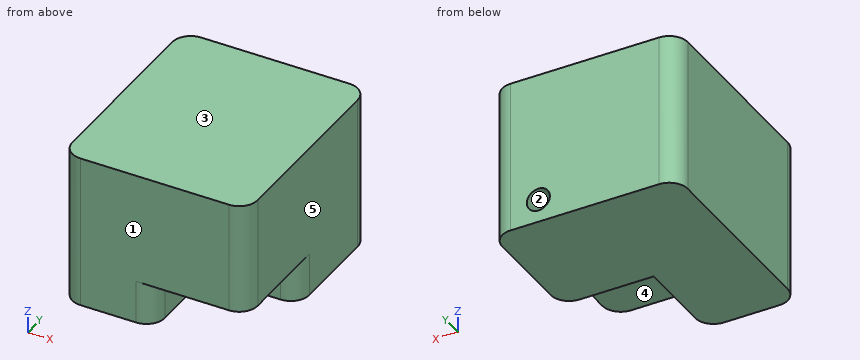
```python
from build123d import *

# Parameters (mm, degrees)
F0_W     = 30
F0_H     = 25
F1_DEPTH = 35
F2_W     = 15
F2_H     = 7
F3_DEPTH = 15
F4_R     = 1.865436
F5_DEPTH = 20.001
F6_R     = 3


with BuildPart() as f1:
    # F0 (on Front) → F1 (new body)
    with BuildSketch(Plane.XZ):
        with Locations((15, -12.5)):
            Rectangle(F0_W, F0_H)
    extrude(amount=F1_DEPTH)

    # F2 (on face) → F3 (cut)
    with BuildSketch(Plane.XZ.offset(35)):
        with Locations((22.5, -21.5)):
            Rectangle(F2_W, F2_H)
    extrude(amount=-F3_DEPTH, mode=Mode.SUBTRACT)

    # F4 (on face) → F5 (cut, through all)
    with BuildSketch(Plane.XZ.offset(20)):
        with Locations((22.5, -21.223269)):
            Circle(F4_R)
    extrude(amount=-F5_DEPTH, mode=Mode.SUBTRACT)

    # F6
    f6_edges = [f1.edges().sort_by_distance(p)[0] for p in [
        (0, -35, -12.5),
        (15, -35, -21.5),
        (30, 0, -12.5),
        (30, -35, -9),
        (30, -20, -21.5),
        (0, 0, -12.5),
    ]]
    fillet(f6_edges, radius=F6_R)


solid = f1.part
```
CAD build for the part. Positions are in the model's coordinates, mm. Face numbers are marked on the shaded views. A direction names the side the tool comes from. Coordinates: 2 decimals unless noted, no trailing zeros. Order: outer loops, then holes, each group sorted by start corner. A loop starts at its lowest first (then second) coordinate and runs counter-clockwise, first axis right, second up.
(1) Drill centre lines: L1, parallel to Z at x = 22.5, y = -6; L2, parallel to Z at x = 23.5, y = -3.5; L3, parallel to Z at x = 15.5, y = -22. Where is each one in solid material? Low to high.
Solution:
L1: z = -25 to -23.09, -19.36 to 0
L2: z = -25 to -22.8, -19.65 to 0
L3: z = -18 to 0
(2) Saw through at D-D, the plane y = -26.5. Write the cut outline in (x, z).
Solution:
outline: (0, -25) - (15, -25) - (15, -18) - (30, -18) - (30, 0) - (0, 0) - close
(3) Saw through at B-B, the plane y = -19. Write the cut outline in (x, z), and give its area (3 significant figures).
Solution:
outline: (0, -25) - (29.24, -25) - (29.24, -18) - (30, -18) - (30, 0) - (0, 0) - close; hole circle Ø3.73 at (22.5, -21.22)
area: 734 mm2
(4) Mould opens along Z. For the marked faces 1, 2 and 3 say: released by +Z, released by -Z, zero draft, split by the parting line, or undercut.
Solution:
face 1: zero draft
face 2: undercut
face 3: released by +Z
(5) Which spindle directions (+Z, -Z, +X, -X, +Y, -Y) get a long thin tool onto all of the face, cutting with end or side? Do the marked faces 4 and 5. Say none if no direction does.
Solution:
face 4: -Z, +X, -Y
face 5: +Z, -Z, +X, +Y, -Y
(6) Saw through at A-A, the plane x = 22.5. Write the cut outline in (y, z).
Solution:
outline: (-35, -18) - (-20, -18) - (-20, -19.36) - (0, -19.36) - (0, 0) - (-35, 0) - close; (-20, -25) - (0, -25) - (0, -23.09) - (-20, -23.09) - close
(7) Pin check, flat tips, straight feed: pin 1 Ø2 at (y, z) = (-26, -21.5) entering from +X; pin 2 Ø3.5 at (x, z) = (23.5, -22.5) entering from -Y. Stop position of each tip, or through.
Solution:
pin 1: stops at x = 15
pin 2: stops at y = -20
(8) Saw through at C-C, the plane x = 25.75. Write the cut outline in (y, z), and give its area (3 significant figures).
Solution:
outline: (-35, -18) - (-20, -18) - (-20, -25) - (0, -25) - (0, 0) - (-35, 0) - close
area: 770 mm2
